Source: CAD feature listing. Evaluate the final solid. Frame: model axes, mm. A direction names the side the tool comes from. Round coordinates to 2 decimals unless told otherwise and drop trailing zeros. Loops run counter-clockwise (first coordinate to the right, second up) from the corner with the lowest first, then second, coordinate; pieces in that order, holes last. Notation, with made-up numbers: M -38.75,-35 L 10.25,-35 A33 cw 10.25,-4 Z; hole C -24,-15 d6. An arc over 180 degrees is marked long. One line per item, written item: value.
from build123d import *

# Parameters (mm, degrees)
BOSS_EXTRUDE1_DEPTH = 15
SHELL1_T            = -2.75
SKETCH2_R           = 2.75
SKETCH2_R_2         = 3.071803615
CUT_EXTRUDE1_DEPTH  = 10
CHAMFER1_SIZE       = 20


with BuildPart() as part:
    # Sketch1 → Boss-Extrude1 (new body)
    with BuildSketch(Plane(origin=(0, 0, 0), x_dir=(1, 0, 0), z_dir=(0, 1, 0))):
        Polygon((-227.5, 100), (-212.5, 100), (-212.5, 7.5), (-80, 7.5), (-80, 27.5), (0, 27.5), (0, 7.5), (0, -7.5), (0, -27.5), (-80, -27.5), (-80, -7.5), (-212.5, -7.5), (-212.5, -60), (-227.5, -60), align=None)
    extrude(amount=BOSS_EXTRUDE1_DEPTH)

    # Shell1
    shell1_openings = [part.faces().sort_by_distance(p)[0] for p in [
        (-113.191678521, 0, -5.46230441),
    ]]
    offset(amount=SHELL1_T, openings=shell1_openings, kind=Kind.INTERSECTION)

    # Sketch2 → Cut-Extrude1 (cut)
    with BuildSketch(Plane(origin=(0, 15, 0), x_dir=(1, 0, 0), z_dir=(0, 1, 0))):
        with Locations(Location((-130, 0, 0), (0, 0, 270))):
            Circle(SKETCH2_R)
        with Locations(Location((-220, 95, 0), (0, 0, 270))):
            Circle(SKETCH2_R)
        with Locations(Location((-220, -55, 0), (0, 0, 270))):
            Circle(SKETCH2_R)
        with Locations(Location((-175, 0, 0), (0, 0, 270))):
            Circle(SKETCH2_R_2)
    extrude(amount=-CUT_EXTRUDE1_DEPTH, mode=Mode.SUBTRACT)

    # Chamfer1
    chamfer1_edges = [part.edges().sort_by_distance(p)[0] for p in [
        (-212.5, 7.5, -7.5),
        (-212.5, 7.5, 7.5),
        (-80, 7.5, -7.5),
        (-80, 7.5, 7.5),
    ]]
    chamfer(chamfer1_edges, length=CHAMFER1_SIZE - 0.0001)  # a hair under: the kernel refuses the full size


solid = part.part
1. Pin query (flat end, axial travel): pin 1 (3 mm diameter, centred on y = 10, z = 39.5, fed in from +X); pin 2 (3.5 mm diameter, centred on x = -174.5, y = 4, fed in from +Z); pin 3 (8 mm diameter, centred on x = -45, y = 3, fed in from +Z). Return the tip coordinate at first contact, or that it passes through.
Report:
pin 1: stops at x = -212.5
pin 2: stops at z = 7.5
pin 3: stops at z = 27.5
2. Section query D-D (z = -95). Return the cut outline in (x, y), and give its area (3 significant figures).
Report:
outline: M -227.5,0 L -224.75,0 L -224.75,12.25 L -222.75,12.25 L -222.75,15 L -227.5,15 Z; M -217.25,12.25 L -215.25,12.25 L -215.25,0 L -212.5,0 L -212.5,15 L -217.25,15 Z
area: 93.5 mm2
3. Section query A-A (x = -130). Return the cut outline in (y, z).
Report:
outline: M 0,-7.5 L 15,-7.5 L 15,-2.75 L 12.25,-2.75 L 12.25,-4.75 L 0,-4.75 Z; M 0,4.75 L 12.25,4.75 L 12.25,2.75 L 15,2.75 L 15,7.5 L 0,7.5 Z
4. Pull-direction query (X, two-part tool) for faces 5 (the face through (-147, 6, -4.75)), 6 (the face through (-212.5, 7, -64)), 7 (the face through (-113, 15, -3)); classes: released by +X, released by -X, zero draft, split by the parting line, or undercut.
Report:
face 5: undercut
face 6: released by +X
face 7: zero draft
5. Ray query, line 1 (X direction, y = 13.65, z = 0); line 2 (Z direction, x = -220, y = 8.5); line 3 (Z direction, x = -46.5, y = 6.5). Return the intervals inside material, ascending. Write a range as [from, to].
Report:
line 1: x = [-227.5, -178.07], [-171.93, -132.75], [-127.25, 0]
line 2: z = [-100, -97.75], [57.75, 60]
line 3: z = [-27.5, -24.75], [24.75, 27.5]
6. Section query B-B (z = 0). Return the cut outline in (x, y), and give its area (3 significant figures).
Report:
outline: M -227.5,0 L -224.75,0 L -224.75,12.25 L -178.07,12.25 L -178.07,15 L -227.5,15 Z; M -171.93,12.25 L -132.75,12.25 L -132.75,15 L -171.93,15 Z; M -127.25,12.25 L -2.75,12.25 L -2.75,0 L 0,0 L 0,15 L -127.25,15 Z
area: 661 mm2
7. Reachability of faces 1 (the face through (-145, 6, 4.75)), 2 (the face through (-202, 7, -17)), 3 (the face through (-219.879, 12.292, -97.747)), 4 (the face through (-203, 7, 18)) from +Z, -Z, +X, -X, +Y, -Y: full face, straight path, thin tool, end or side. Return the list, or none.
Report:
face 1: -Y
face 2: -Z, +Y, -Y
face 3: +Y
face 4: +Z, +Y, -Y
